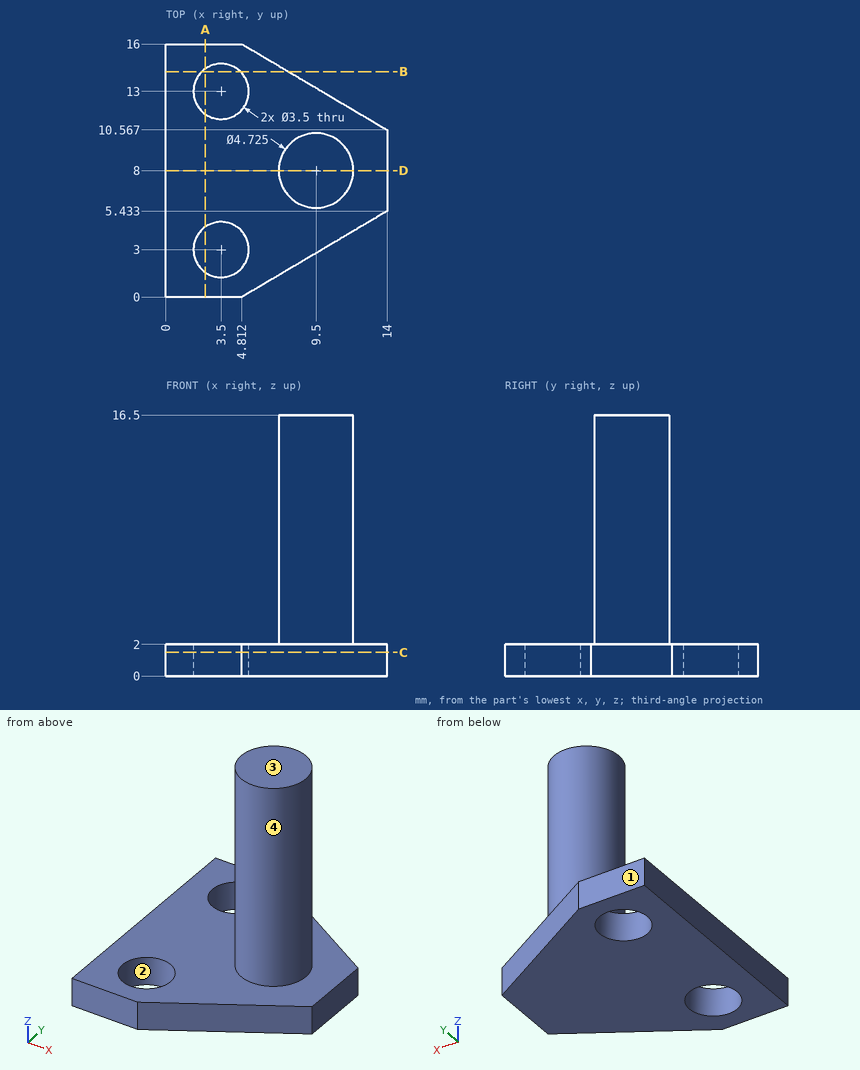
Could you check a few things on this drawing? It's one solid part, dimensions in mm from its lowest x, y, z. Round coordinates to 2 decimals unless told otherwise and drop trailing zeros. Order: outer loops, then holes, each group sorted by start corner. A loop starts at its lowest first (then second) coordinate and runs counter-clockwise, first axis right, second up. Notation, with made-up numbers: M 21,-37 L 29,-37 A6 ccw 29,-27 Z; hole C 65.5,52 d5. An arc over 180 degrees is marked long. One line per question, with ' | ' between items. Start each with the question number.
(1) Thinking about a two-plate mould opening in Y: for the marked faces 1, 2, 3 and 4, which applies, +Y half, -Y half, draft (parallel to the pull), parting line (faces both ways), or undercut?
(2) Suppose I cut it at B-B on y = 14.25. List the corners of the cut face in (x, z) for me (1 decimal).
(3) Suppose I cut it at D-D on y = 8. List the corners of the cut face in (x, z) for me.
(4) Suppose I cut it at A-A on x = 2.5. List the corners of the cut face in (y, z) for me, then the cut area to 3 significant figures.
(5) For P1, Ø8, axis at y = 10.5, z = 13, coming from the +X side; P2, Ø1, axis at x = 6, y = 14, coming from the +Z side; P3, Ø1.5, axis at x = 7, z = 13.5, coming from the -Y side; P4, Ø5, axis at x = 1.5, y = 8.5, coming from the -Z side, each with a flat end and sliding along its axis, tell me the tip position at first contact or that it passes through.
(6) Suppose I cut it at C-C on z = 1.5. List the corners of the cut face in (x, y) for me.
(7) Please list where these lines run through material, in increasing order: line 1 along Y through (x, z) = (3.5, 0.55); line 2 along Z through (x, y) = (10.25, 4); line 3 along X through (y, z) = (7, 3).
Geometry results:
1) face 1: +Y half | face 2: undercut | face 3: draft | face 4: parting line
2) outline: M 0,0 L 2.3,0 L 2.3,2 L 0,2 Z; M 4.7,0 L 7.8,0 L 7.8,2 L 4.7,2 Z
3) outline: M 0,0 L 14,0 L 14,2 L 11.86,2 L 11.86,16.5 L 7.14,16.5 L 7.14,2 L 0,2 Z
4) outline: M 0,0 L 1.56,0 L 1.56,2 L 0,2 Z; M 4.44,0 L 11.56,0 L 11.56,2 L 4.44,2 Z; M 14.44,0 L 16,0 L 16,2 L 14.44,2 Z | area: 20.5 mm²
5) P1: x = 11.86 | P2: z = 2 | P3: y = 6.41 | P4: z = 0
6) outline: M 0,0 L 4.81,0 L 14,5.43 L 14,10.57 L 4.81,16 L 0,16 Z; hole C 3.5,3 d3.5; hole C 3.5,13 d3.5
7) line 1: 0 to 1.25, 4.75 to 11.25, 14.75 to 16 | line 2: 0 to 2 | line 3: 7.36 to 11.64
